Read the model definition and answer for the solid it produces. Units are mm, in the model's axes. A direction names the side the tool comes from. Give positions to 0.01 mm unless a question says otherwise; leave off trailing zeros. Order: outer loops, then holes, each group sorted by start corner. A loop starts at its lowest first (then second) coordinate and runs counter-clockwise, first axis right, second up. Notation, with made-up numbers: (-40, 9) -> (-13, 9) arc R25 cw to (-13, 26) -> close; hole circle Ø5 at (-35, 27.25). An arc over 180 degrees is marked (long way). Use one line per item in the form item = value.
```python
from build123d import *

# Parameters (mm, degrees)
CROQUIS1_W              = 190.5
CROQUIS1_H              = 914.4
SALIENTE_EXTRUIR1_DEPTH = 95.25
CROQUIS2_W              = 149.86
CROQUIS2_H              = 152.4
CORTAR_EXTRUIR1_DEPTH   = 177.8
CORTAR_EXTRUIR3_START   = 152.4
CROQUIS3_W              = 149.86
CROQUIS3_H              = 165.1
CORTAR_EXTRUIR3_DEPTH   = 457.2


with BuildPart() as part:
    # Croquis1 → Saliente-Extruir1 (new body, symmetric)
    with BuildSketch(Plane.XY):
        Rectangle(CROQUIS1_W, CROQUIS1_H)
    extrude(amount=SALIENTE_EXTRUIR1_DEPTH, both=True)

    # Croquis2 → Cortar-Extruir1 (cut)
    with BuildSketch(Plane.XY.offset(95.25)):
        with Locations((1.27, 304.8)):
            Rectangle(CROQUIS2_W, CROQUIS2_H)
        with Locations((1.27, 0)):
            Rectangle(CROQUIS2_W, CROQUIS2_H)
        with Locations((1.27, -304.8)):
            Rectangle(CROQUIS2_W, CROQUIS2_H)
    extrude(amount=-CORTAR_EXTRUIR1_DEPTH, mode=Mode.SUBTRACT)

    # Croquis3 → Cortar-Extruir3 (cut)
    with BuildSketch(Plane.XZ.offset(-381).offset(CORTAR_EXTRUIR3_START)):
        with Locations((1.27, 0)):
            Rectangle(CROQUIS3_W, CROQUIS3_H)
    extrude(amount=CORTAR_EXTRUIR3_DEPTH, mode=Mode.SUBTRACT)


solid = part.part
```
Item 1: Given pin 1 Ø1.5 at (x, y) = (-35, -267) entering from +Z, flat-ended and moving along its own axis, determine where the tip first touches the part or whether it passes through.
Checks:
pin_1 = -82.55
Item 2: The part is cut by section A-A on x = -42. Give the vertices of the cut face in (y, z), and give its area (3 significant figures).
Checks:
outline = (-457.2, -95.25) -> (457.2, -95.25) -> (457.2, 95.25) -> (381, 95.25) -> (381, -82.55) -> (-381, -82.55) -> (-381, 95.25) -> (-457.2, 95.25) -> close; (-228.6, 82.55) -> (-76.2, 82.55) -> (-76.2, 95.25) -> (-228.6, 95.25) -> close; (76.2, 82.55) -> (228.6, 82.55) -> (228.6, 95.25) -> (76.2, 95.25) -> close
area = 42,600 mm²
Item 3: Determine the mould class of faces 1 (the flat face through (-95.25, -6, 1)), 2 (the flat face through (0, 5, -82.55)), 3 (the flat face through (-1, -457.2, 1)) for opening direction X: +X half, -X half, draft (parallel to the pull), parting line (faces both ways), or undercut.
Checks:
face_1 = -X half
face_2 = undercut
face_3 = draft
Item 4: The part is cut by section C-C on z = -40. Give the vertices of the cut face in (x, y), and give its area (3 significant figures).
Checks:
outline = (-95.25, -457.2) -> (95.25, -457.2) -> (95.25, 457.2) -> (-95.25, 457.2) -> close; hole (-73.66, -381) -> (76.2, -381) -> (76.2, 381) -> (-73.66, 381) -> close
area = 60,000 mm²
Item 5: Which of the six approach directions +Z, -Z, +X, -X, +Y, -Y give full straight-line access (tool end or side, diameter ignored) to faces 4 (the flat face through (-73.66, -5, 8)), 5 (the flat face through (0, 381, 8)), 6 (the flat face through (83, 6, 95.25))?
Checks:
face_4 = none
face_5 = +Z
face_6 = +Z, +X, -X, +Y, -Y
Item 6: Straight lines are drawn through the part: L1, parallel to Y at x = 17, z = 84; L2, parallel to Z at x = -11, y = 156; L3, parallel to Y at x = -34.5, z = -16. For each, find the intervals that lie inside material, in ascending order. Write a range as from..to.
Checks:
L1 = -457.2..-381, -228.6..-76.2, 76.2..228.6, 381..457.2
L2 = -95.25..-82.55, 82.55..95.25
L3 = -457.2..-381, 381..457.2
Item 7: The part is cut by section D-D on y = 304. Give the vertices of the cut face in (x, z).
Checks:
outline = (-95.25, -95.25) -> (95.25, -95.25) -> (95.25, 95.25) -> (76.2, 95.25) -> (76.2, -82.55) -> (-73.66, -82.55) -> (-73.66, 95.25) -> (-95.25, 95.25) -> close
Item 8: The part is cut by section B-B on y = 137. Give the vertices of the cut face in (x, z).
Checks:
outline = (-95.25, -95.25) -> (95.25, -95.25) -> (95.25, 95.25) -> (-95.25, 95.25) -> close; hole (-73.66, -82.55) -> (76.2, -82.55) -> (76.2, 82.55) -> (-73.66, 82.55) -> close
